Source: CAD feature listing. Evaluate the final solid. Frame: model axes, mm. Give positions to 0.01 mm unless a question says otherwise; leave off trailing zeros. Write each loop counter-clockwise with the first axis right and the second up, starting at its lowest first coordinate (ties: lowest second). Pieces come first, ordered by that corner, then holes.
```python
from build123d import *

# Parameters (mm, degrees)
F0_W          = 87.8805932263
F0_H          = 80
F1_DEPTH      = 80
F2_R          = 13.7808794965
F3_DEPTH      = 25
F4_R          = 13.7808794965
F7_DEPTH      = 25
F5_R          = 13.7808794965
F8_DEPTH      = 25
F6_R          = 13.7808794965
F9_DEPTH      = 105.001
F10_R         = 5
F11_T1_DEPTH  = 87.5
F11_S5_W      = 5
F11_S5_H      = 5
F11_T6_DEPTH  = 5
F11_S11_W     = 5
F11_S11_H     = 5
F11_T12_DEPTH = 5
F11_S17_W     = 5
F11_S17_H     = 5
F11_T18_DEPTH = 5
F11_S23_W     = 5
F11_S23_H     = 5
F11_T24_DEPTH = 5


# Not quite as in the source:
# - a fillet or chamfer that OpenCascade refuses, or shapes differently, is made with other operations: its cross-section is extruded or revolved along the edge and cut away or added


with BuildPart() as f1:
    # F0 (on Top) → F1 (new body)
    with BuildSketch(Plane.XY):
        Rectangle(F0_W, F0_H)
    extrude(amount=F1_DEPTH)

    # F2 (on face) → F3 (join)
    with BuildSketch(Plane.XY.offset(80)):
        Circle(F2_R)
    extrude(amount=F3_DEPTH)

    # F4 (on face) → F7 (cut)
    with BuildSketch(Plane.XY.offset(105)):
        Circle(F4_R)
    extrude(amount=-F7_DEPTH, mode=Mode.SUBTRACT)

    # F5 (on face) → F8 (cut)
    with BuildSketch(Plane.XY):
        Circle(F5_R)
    extrude(amount=-F8_DEPTH, mode=Mode.SUBTRACT)

    # F6 (on face) → F9 (cut, through all)
    with BuildSketch(Plane.XY.offset(105)):
        Circle(F6_R)
    extrude(amount=-F9_DEPTH, mode=Mode.SUBTRACT)

    # F10
    f10_edges = [f1.edges().sort_by_distance(p)[0] for p in [
        (0, 40, 80),
        (43.940297, 0, 80),
        (-43.940297, 0, 80),
        (0, -40, 80),
        (-13.780879, 0, 80),
    ]]
    fillet(f10_edges, radius=F10_R)

    # F11: fillet of radius 5 on 15 edges, made by hand

    # F11_s2 → F11_t1 (cut)
    with BuildSketch(Plane.XY.offset(-12.5)):
        with BuildLine():
            ThreePointArc((-43.9402966131, -35), (-42.4758305191, -38.5355339059), (-38.9402966131, -40))
            Line((-38.9402966131, -40), (-43.9402966131, -40))
            Line((-43.9402966131, -40), (-43.9402966131, -35))
        make_face()
        with BuildLine():
            ThreePointArc((43.9402966131, -35), (42.4758305191, -38.5355339059), (38.9402966131, -40))
            Line((38.9402966131, -40), (43.9402966131, -40))
            Line((43.9402966131, -40), (43.9402966131, -35))
        make_face()
        with BuildLine():
            ThreePointArc((-38.9402966131, 40), (-42.4758305191, 38.5355339059), (-43.9402966131, 35))
            Line((-43.9402966131, 35), (-43.9402966131, 40))
            Line((-43.9402966131, 40), (-38.9402966131, 40))
        make_face()
        with BuildLine():
            ThreePointArc((38.9402966131, 40), (42.4758305191, 38.5355339059), (43.9402966131, 35))
            Line((43.9402966131, 35), (43.9402966131, 40))
            Line((43.9402966131, 40), (38.9402966131, 40))
        make_face()
    extrude(amount=F11_T1_DEPTH, mode=Mode.SUBTRACT)


with BuildPart() as f11_tool4:
    # F11_s5 → F11_t6 (new body)
    with BuildSketch(Plane.XZ.offset(-35)):
        with Locations((41.4402966131, 77.5)):
            Rectangle(F11_S5_W, F11_S5_H)
    extrude(amount=-F11_T6_DEPTH)

    # F11_s7 → F11_t8 (revolve, cut)
    with BuildSketch(Plane(origin=(38.9402966131, 35, 75), x_dir=(-0.7071067812, 0, -0.7071067812), z_dir=(0.7071067812, 0, -0.7071067812))):
        with BuildLine():
            ThreePointArc((0, -5), (5, 0), (0, 5))
            Line((0, 5), (0, -5))
        make_face()
    revolve(axis=Axis((38.9402966131, 35, 75), (0, 1, 0)), mode=Mode.SUBTRACT)


with BuildPart() as f1_1:
    add(f1.part)

    # F11_t3: cut F11_tool4
    add(f11_tool4.part, mode=Mode.SUBTRACT)


with BuildPart() as f11_tool10:
    # F11_s11 → F11_t12 (new body)
    with BuildSketch(Plane.XZ.offset(-35)):
        with Locations((-41.4402966131, 77.5)):
            Rectangle(F11_S11_W, F11_S11_H)
    extrude(amount=-F11_T12_DEPTH)

    # F11_s13 → F11_t14 (revolve, cut)
    with BuildSketch(Plane(origin=(-38.9402966131, 35, 75), x_dir=(0.7071067812, 0, -0.7071067812), z_dir=(0.7071067812, 0, 0.7071067812))):
        with BuildLine():
            ThreePointArc((0, -5), (5, 0), (0, 5))
            Line((0, 5), (0, -5))
        make_face()
    revolve(axis=Axis((-38.9402966131, 35, 75), (0, 1, 0)), mode=Mode.SUBTRACT)


with BuildPart() as f1_2:
    add(f1_1.part)

    # F11_t9: cut F11_tool10
    add(f11_tool10.part, mode=Mode.SUBTRACT)


with BuildPart() as f11_tool16:
    # F11_s17 → F11_t18 (new body)
    with BuildSketch(Plane.YZ.offset(38.9402966131)):
        with Locations((-37.5, 77.5)):
            Rectangle(F11_S17_W, F11_S17_H)
    extrude(amount=F11_T18_DEPTH)

    # F11_s19 → F11_t20 (revolve, cut)
    with BuildSketch(Plane(origin=(38.9402966131, -35, 75), x_dir=(0, 0.7071067812, -0.7071067812), z_dir=(0, -0.7071067812, -0.7071067812))):
        with BuildLine():
            ThreePointArc((0, -5), (5, 0), (0, 5))
            Line((0, 5), (0, -5))
        make_face()
    revolve(axis=Axis((38.9402966131, -35, 75), (1, 0, 0)), mode=Mode.SUBTRACT)


with BuildPart() as f1_3:
    add(f1_2.part)

    # F11_t15: cut F11_tool16
    add(f11_tool16.part, mode=Mode.SUBTRACT)


with BuildPart() as f11_tool22:
    # F11_s23 → F11_t24 (new body)
    with BuildSketch(Plane.YZ.offset(-38.9402966131)):
        with Locations((-37.5, 77.5)):
            Rectangle(F11_S23_W, F11_S23_H)
    extrude(amount=-F11_T24_DEPTH)

    # F11_s25 → F11_t26 (revolve, cut)
    with BuildSketch(Plane(origin=(-38.9402966131, -35, 75), x_dir=(0, 0.7071067812, -0.7071067812), z_dir=(0, 0.7071067812, 0.7071067812))):
        with BuildLine():
            ThreePointArc((0, -5), (5, 0), (0, 5))
            Line((0, 5), (0, -5))
        make_face()
    revolve(axis=Axis((-38.9402966131, -35, 75), (-1, 0, 0)), mode=Mode.SUBTRACT)


with BuildPart() as f1_4:
    add(f1_3.part)

    # F11_t21: cut F11_tool22
    add(f11_tool22.part, mode=Mode.SUBTRACT)


solid = f1_4.part
```
1. Line query: L1, parallel to Y at x = 0, z = 45.5; L2, parallel to Y at x = -3, z = 63; L3, parallel to Z at x = -17, y = -1. Output: solid intervals per line, ascending.
2. Cut plane C-C, the plane z = 59.5. Return the cut outline in (x, y), then the cut area to 3 significant figures.
3. Cut plane A-A, the plane y = 0. Return the cut outline in (x, z), then the cut area to 3 significant figures.
4. Mould query, pull axis X, two halves, no side actions, for faces 1 (the cylindrical face through (42.44, 38.57, 36.98)), 2 (the cylindrical face through (-10.936, -8.385, 38.025)), 3 (the cylindrical face through (1, 39, 78)), 4 (the cylindrical face through (-42.44, 38.57, 36.98)). Classes: +X half, -X half, draft (parallel to the pull), parting line (faces both ways), or undercut.
5. Cut plane B-B, the plane x = 0. Return the cut outline in (y, z).
Response values:
1. L1: y = -40 to -13.78, 13.78 to 40
1. L2: y = -40 to -13.45, 13.45 to 40
1. L3: z = 0 to 79.68
2. outline: (-43.94, -35) arc R5 ccw to (-38.94, -40) - (38.94, -40) arc R5 ccw to (43.94, -35) - (43.94, 35) arc R5 ccw to (38.94, 40) - (-38.94, 40) arc R5 ccw to (-43.94, 35) - close; hole circle Ø27.56 at (0, 0)
2. area: 6,410 mm2
3. outline: (-43.94, 0) - (-13.78, 0) - (-13.78, 75) arc R5 ccw to (-18.78, 80) - (-38.94, 80) arc R5 ccw to (-43.94, 75) - close; (13.78, 0) - (43.94, 0) - (43.94, 75) arc R5 ccw to (38.94, 80) - (18.78, 80) arc R5 ccw to (13.78, 75) - close
3. area: 4,800 mm2
4. face 1: +X half
4. face 2: undercut
4. face 3: draft
4. face 4: -X half
5. outline: (-40, 0) - (-13.78, 0) - (-13.78, 75) arc R5 ccw to (-18.78, 80) - (-35, 80) arc R5 ccw to (-40, 75) - close; (13.78, 0) - (40, 0) - (40, 75) arc R5 ccw to (35, 80) - (18.78, 80) arc R5 ccw to (13.78, 75) - close
